Geometry check sheet. Reference: the model listing, model coordinates, mm. Face numbers are marked on the shaded views. A direction names the side the tool comes from. Give positions to 0.01 mm unless a question says otherwise; leave off trailing zeros. Loops run counter-clockwise (first coordinate to the right, second up) from the corner with the lowest first, then second, coordinate; pieces in that order, holes last. Notation, with made-up numbers: (11, -17.5) -> (18, -17.5) arc R10 cw to (18, -8.5) -> close; hole circle Ø9 at (60, 3.25). An arc over 180 degrees is marked (long way). One line per question, with ' | ' between items.
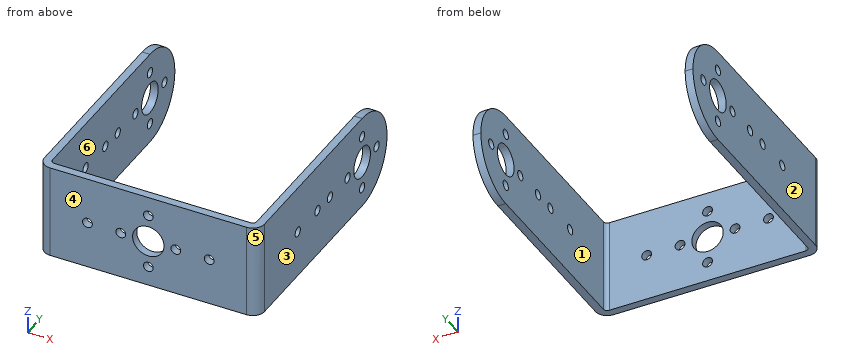
from build123d import *

# Parameters (mm, degrees)
T_LE_DE_BASE_PLI_E1_DEPTH       = 12
ENL_V_START                     = -56
ENL_V_MAT_EXTRU_1_DEPTH         = 56
DIAM_TRE_DU_PER_AGE_8_0_8_1_D   = 8
DIAM_TRE_DU_PER_AGE_2_5_2_5_1_D = 2.5
DIAM_TRE_DU_PER_AGE_8_0_8_2_D   = 8
DIAM_TRE_DU_PER_AGE_2_5_2_5_2_D = 2.5


# Read off the part's stored shape, not the designer's step: Enlèv. mat.-Extru.1
# Sheet-metal steps are written as plain solids
with BuildPart() as part:
    # Esquisse1 → Tôle de base pliée1 (new, symmetric)
    with BuildSketch(Plane.XY):
        with BuildLine():
            Line((-28, 62), (-28, 3))
            ThreePointArc((-28, 3), (-27.121320344, 0.878679656), (-25, 0))
            Line((-25, 0), (25, 0))
            ThreePointArc((25, 0), (27.121320344, 0.878679656), (28, 3))
            Line((28, 3), (28, 62))
            Line((28, 62), (26, 62))
            Line((26, 62), (26, 3))
            ThreePointArc((26, 3), (25.707106781, 2.292893219), (25, 2))
            Line((25, 2), (-25, 2))
            ThreePointArc((-25, 2), (-25.707106781, 2.292893219), (-26, 3))
            Line((-26, 3), (-26, 62))
            Line((-26, 62), (-28, 62))
        make_face()
    extrude(amount=T_LE_DE_BASE_PLI_E1_DEPTH, both=True)

    # Enlèv. mat.-Extru.1 outline → Enlèv. mat.-Extru.1 (cut)
    with BuildSketch(Plane(origin=(28, 0, 0), x_dir=(0, 0, -1), z_dir=(1, 0, 0)).offset(ENL_V_START)):
        with BuildLine():
            ThreePointArc((-12, 50), (-8.485281374, 58.485281374), (0, 62))
            Line((0, 62), (-12, 62))
            Line((-12, 62), (-12, 50))
        make_face()
        with BuildLine():
            ThreePointArc((0, 62), (8.485281374, 58.485281374), (12, 50))
            Line((12, 50), (12, 62))
            Line((12, 62), (0, 62))
        make_face()
    extrude(amount=ENL_V_MAT_EXTRU_1_DEPTH, mode=Mode.SUBTRACT)

    # Diamètre du perçage Ø8.0 (8)1 (through all)
    with Locations(Plane(origin=(28, 0, 0), x_dir=(0, 0, -1), z_dir=(1, 0, 0))):
        with Locations((0, 50)):
            Hole(DIAM_TRE_DU_PER_AGE_8_0_8_1_D / 2)

    # Diamètre du perçage Ø2.5 (2.5)1 (through all)
    with Locations(Plane(origin=(28, 0, 0), x_dir=(0, 0, -1), z_dir=(1, 0, 0))):
        with Locations((0, 57), (7, 50), (0, 43), (-7, 50), (0, 34.5), (0, 28.5), (0, 19)):
            Hole(DIAM_TRE_DU_PER_AGE_2_5_2_5_1_D / 2)

    # Diamètre du perçage Ø8.0 (8)2 (through all)
    with Locations(Plane(origin=(0, 2, 0), x_dir=(1, 0, 0), z_dir=(0, 1, 0))):
        with Locations((0, 0)):
            Hole(DIAM_TRE_DU_PER_AGE_8_0_8_2_D / 2)

    # Diamètre du perçage Ø2.5 (2.5)2 (through all)
    with Locations(Plane(origin=(0, 2, 0), x_dir=(1, 0, 0), z_dir=(0, 1, 0))):
        with Locations((0, 7), (7, 0), (0, -7), (-7, 0), (-15.5, 0), (15.5, 0)):
            Hole(DIAM_TRE_DU_PER_AGE_2_5_2_5_2_D / 2)


solid = part.part
Item 1: Sectioned sample at D-D (z = 3). Record the cut outline in (x, y).
Result:
outline: (-28, 3) arc R3 ccw to (-25, 0) -> (-2.65, 0) -> (-2.65, 2) -> (-25, 2) arc R1 cw to (-26, 3) -> (-26, 47.35) -> (-28, 47.35) -> close; (-28, 52.65) -> (-26, 52.65) -> (-26, 61.62) -> (-28, 61.62) -> close; (2.65, 0) -> (25, 0) arc R3 ccw to (28, 3) -> (28, 47.35) -> (26, 47.35) -> (26, 3) arc R1 cw to (25, 2) -> (2.65, 2) -> close; (26, 52.65) -> (28, 52.65) -> (28, 61.62) -> (26, 61.62) -> close
Item 2: Depth check by flat-ended pin: pin 1 Ø3 at (x, z) = (0, -7) entering from +Y. Enter the tip coordinate at first touch or a pass-through.
Result:
pin 1: y = 2
Item 3: Set-up check for the marked faces 5 and 6: record each of +Z, -Z, +X, -X, +Y, -Y from which the full face is reachable in a straight line by a thin tool's end or side.
Result:
face 5: +Z, -Z, +X, -Y | face 6: +Z, -Z, +Y
Item 4: Sectioned sample at A-A (x = -15.5). Record the cut outline in (y, z), plus the area to 3 significant figures.
Result:
outline: (0, -12) -> (2, -12) -> (2, -1.25) -> (0, -1.25) -> close; (0, 1.25) -> (2, 1.25) -> (2, 12) -> (0, 12) -> close | area: 43.0 mm2
Item 5: Sectioned sample at C-C (x = 0). Record the cut outline in (y, z).
Result:
outline: (0, -12) -> (2, -12) -> (2, -8.25) -> (0, -8.25) -> close; (0, -5.75) -> (2, -5.75) -> (2, -4) -> (0, -4) -> close; (0, 4) -> (2, 4) -> (2, 5.75) -> (0, 5.75) -> close; (0, 8.25) -> (2, 8.25) -> (2, 12) -> (0, 12) -> close
Item 6: Scan lines: probe 1 along X at (y, z) = (30.5, 10.25); probe 2 along Z at (x, y) = (-7, 1.5); probe 3 along Y at (x, z) = (-19.5, -3.25). Record each from-to range of solid material in increasing order.
Result:
probe 1: -28 to -26, 26 to 28 | probe 2: -12 to -1.25, 1.25 to 12 | probe 3: 0 to 2
Item 7: Release check for a two-part mould opening along X. For the marked faces 1, 2, 3 and 4 record: pulls with the +X half, pulls with the -X half, needs draft (parallel to the pull), parting line crosses it, or undercut.
Result:
face 1: undercut | face 2: pulls with the -X half | face 3: pulls with the +X half | face 4: needs draft
Item 8: Sectioned sample at B-B (y = 28.5). Record the cut outline in (x, z).
Result:
outline: (-28, -12) -> (-26, -12) -> (-26, -1.25) -> (-28, -1.25) -> close; (-28, 1.25) -> (-26, 1.25) -> (-26, 12) -> (-28, 12) -> close; (26, -12) -> (28, -12) -> (28, -1.25) -> (26, -1.25) -> close; (26, 1.25) -> (28, 1.25) -> (28, 12) -> (26, 12) -> close
